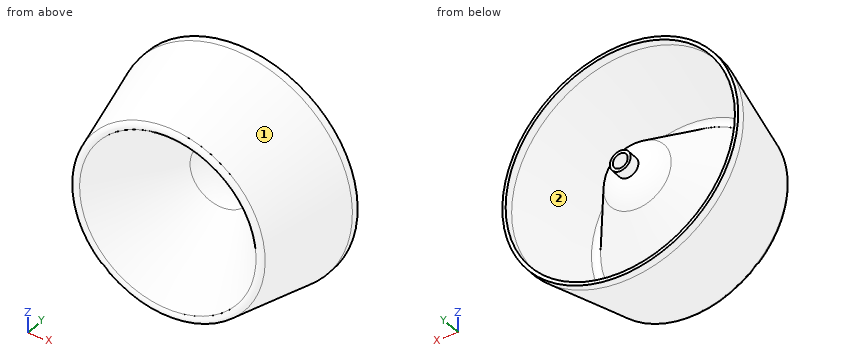
```python
from build123d import *


with BuildPart() as part:
    # Sketch1 → Revolve7 (revolve)
    with BuildSketch(Plane(origin=(0, 0, 0), x_dir=(0, 0, -1), z_dir=(1, 0, 0))):
        with BuildLine():
            Line((-59.148631637, -32.404719831), (-21.068373541, 19.926718309))
            ThreePointArc((-21.068373541, 19.926718309), (-14.017788653, 26.011562826), (-5, 28.338700093))
            Line((-5, 28.338700093), (-5, 37.743055381))
            Line((-5, 37.743055381), (-7, 37.743055381))
            Line((-7, 37.743055381), (-7, 30.208100681))
            ThreePointArc((-7, 30.208100681), (-15.803114649, 27.310289813), (-22.685536518, 21.103486724))
            Line((-22.685536518, 21.103486724), (-58.176080505, -27.669061048))
            ThreePointArc((-58.176080505, -27.669061048), (-61.205332633, -28.842577937), (-63.526904277, -26.570174926))
            Line((-63.526904277, -26.570174926), (-76.841870349, 31.885910778))
            Line((-76.841870349, 31.885910778), (-76.841870349, 37.743055381))
            Line((-76.841870349, 37.743055381), (-79.058926618, 37.743055381))
            Line((-79.058926618, 37.743055381), (-79.058926618, 32.613945898))
            Line((-79.058926618, 32.613945898), (-64.499455409, -31.305833709))
            ThreePointArc((-64.499455409, -31.305833709), (-62.177883765, -33.578236719), (-59.148631637, -32.404719831))
        make_face()
    revolve(axis=Axis((0, 0, 0), (0, -1, 0)))


solid = part.part
```
Model file for the job. Use its own axes, mm. Face numbers are marked on the shaded views. Coordinates: 2 decimals unless noted, no trailing zeros. Use a Markdown table: item, result. Add a question column.
Item 1: Drill centre lines: line 1 along Z through (x, y) = (0, 35); line 2 along Z through (x, y) = (2.5, -0.5). Where is each one in solid material? Low to high.
Item 2: Drop flat-ended pins along their axis: pin 1 (1.5 mm diameter, centred on y = -7, z = -48.5, fed in from +X); pin 2 (10 mm diameter, centred on y = -19, z = -7, fed in from +X); pin 3 (3 mm diameter, centred on y = -6, z = -39, fed in from -X). Give the stop position or say it passes through.
Item 3: Two-plate mould, pull along X, no slides. Class the marked faces 1 and 2: pulls with the +X half, pulls with the -X half, needs draft (parallel to the pull), parting line crosses it, or undercut.
A:
| question | item | result |
|---|---|---|
| 1 | line 1 | z = -79.06 to -76.84, -7 to -5, 5 to 7, 76.84 to 79.06 |
| 1 | line 2 | z = -71.47 to -69.42, -38.32 to -35.85, 35.85 to 38.32, 69.42 to 71.47 |
| 2 | pin 1 | stops at x = 51.27 |
| 2 | pin 2 | stops at x = 68.17 |
| 2 | pin 3 | stops at x = -59.5 |
| 3 | face 1 | parting line crosses it |
| 3 | face 2 | undercut |
